```python
from build123d import *

# Parameters (mm, degrees)
BOSS_EXTRUDE1_DEPTH = 250.825
SHELL1_T            = -1.5875


with BuildPart() as part:
    # Sketch1 → Boss-Extrude1 (new body)
    with BuildSketch(Plane.XY):
        Polygon((0, 0), (0, 404.8125), (352.425, 404.8125), (454.575413377, 302.662086623), (454.575413377, -279.4), (313.287913377, -420.6875), (313.287913377, 0), align=None)
    extrude(amount=-BOSS_EXTRUDE1_DEPTH)

    # Shell1
    shell1_openings = [part.faces().sort_by_distance(p)[0] for p in [
        (313.287913377, -210.34375, -125.4125),
        (156.643956689, 0, -125.4125),
    ]]
    offset(amount=SHELL1_T, openings=shell1_openings, kind=Kind.INTERSECTION)


solid = part.part
```
Could you check a few things on this model? Use its own coordinates, in mm. A direction names the side the tool comes from. Round coordinates to 2 decimals unless told otherwise and drop trailing zeros. Loops run counter-clockwise (first coordinate to the right, second up) from the corner with the lowest first, then second, coordinate; pieces in that order, holes last. Notation, with made-up numbers: M 6,-10.5 L 13,-10.5 A13 cw 13,12.5 Z; hole C -14.75,43 d9. An arc over 180 degrees is marked long. Answer as CSV lines item,"result".
1) Imagine slicing it at D-D on x = 393.5. List the corners of the cut face in (y, z) for me (1 decimal).
From the geometry:
outline,"M -340.5,-250.8 L 363.7,-250.8 L 363.7,0 L -340.5,0 Z; hole M -338.2,-249.2 L 361.5,-249.2 L 361.5,-1.6 L -338.2,-1.6 Z"
2) For pin 1 Ø2 at (x, z) = (172.5, -50.5) entering from -Y (3 decimals); pin 2 Ø3 at (y, z) = (-170.5, -152) entering from -X, each with a flat end and sliding along its axis, tell me the tip position at first contact or that it passes through.
From the geometry:
pin 1,"y = 403.225"
pin 2,"x = 452.99"
3) Imagine slicing it at A-A on y = -49. List the corners of the cut face in (x, z) for me (1 decimal).
From the geometry:
outline,"M 313.3,-250.8 L 454.6,-250.8 L 454.6,0 L 313.3,0 L 313.3,-1.6 L 453,-1.6 L 453,-249.2 L 313.3,-249.2 Z"
4) If I drill on probe 1 along Z at (x, y) = (115, 173) (1 decimal); probe 2 along X at (y, z) = (199.5, -178.5); probe 3 along Y at (x, z) = (27.5, -169.5) (1 decimal), over which ranges is the centre line in solid material (lowest first)?
From the geometry:
probe 1,"-250.8 to -249.2, -1.6 to 0"
probe 2,"0 to 1.59, 452.99 to 454.58"
probe 3,"403.2 to 404.8"
5) Imagine slicing it at B-B on x = 92. List the corners of the cut face in (y, z) for me (1 decimal).
From the geometry:
outline,"M 0,-250.8 L 404.8,-250.8 L 404.8,0 L 0,0 L 0,-1.6 L 403.2,-1.6 L 403.2,-249.2 L 0,-249.2 Z"
6) Imagine slicing it at C-C on y = 113. List the corners of the cut face in (x, z) for me (1 decimal).
From the geometry:
outline,"M 0,-250.8 L 454.6,-250.8 L 454.6,0 L 0,0 Z; hole M 1.6,-249.2 L 453,-249.2 L 453,-1.6 L 1.6,-1.6 Z"
7) We'd pull the mould along Z, two halves only. Please class faces 1 (the flat face through (452.988, 16, -124)), 2 (the flat face through (281, 90, -250.825)), 3 (the flat face through (281, 89, -249.237)), 4 (the flat face through (402.79, 354.45, -123.66)): released by +Z, released by -Z, zero draft, split by the parting line, or undercut.
From the geometry:
face 1,"undercut"
face 2,"released by -Z"
face 3,"undercut"
face 4,"zero draft"
8) Which directions (+Z, -Z, +X, -X, +Y, -Y) give clear straight access to the entire face, cutting with the end or side of a thin tool? Please do faces 5 (the flat face through (384.12, -347.61, -123.68)), 6 (the flat face through (0, 200, -124)), 7 (the flat face through (1.588, 199, -124)), 8 (the flat face through (281, 89, -1.588)).
From the geometry:
face 5,"-X"
face 6,"+Z, -Z, -X, +Y, -Y"
face 7,"-Y"
face 8,"none"
